Input: part model. Units: mm. Frame: model coordinates. A direction names the side the tool comes from. Round coordinates to 2 decimals unless told otherwise and drop trailing zeros. Loops run counter-clockwise (first coordinate to the right, second up) from the corner with the lowest first, then second, coordinate; pieces in that order, holes last. Notation, with made-up numbers: (-3, 62) -> (16, 62) arc R25 ccw to (16, 74) -> close; hole circle Ø3 at (9.5, 46.5). An arc over 180 degrees is marked (long way). Answer as a JSON object with one key per item and string values.
```python
from build123d import *

# Parameters (mm, degrees)
F1_DEPTH = 550
F2_R     = 6.25
F3_DEPTH = 80.001
F5_DEPTH = 80.001


with BuildPart() as f1:
    # F0 (on Front) → F1 (new body, symmetric)
    with BuildSketch(Plane.XZ):
        with BuildLine():
            ThreePointArc((40, 30), (37.071068, 37.071068), (30, 40))
            Line((30, 40), (-30, 40))
            ThreePointArc((-30, 40), (-37.071068, 37.071068), (-40, 30))
            Line((-40, 30), (-40, -30))
            ThreePointArc((-40, -30), (-37.071068, -37.071068), (-30, -40))
            Line((-30, -40), (30, -40))
            ThreePointArc((30, -40), (37.071068, -37.071068), (40, -30))
            Line((40, -30), (40, 30))
        make_face()
        with BuildLine():
            ThreePointArc((30, 35), (33.535534, 33.535534), (35, 30))
            Line((35, 30), (35, -30))
            ThreePointArc((35, -30), (33.535534, -33.535534), (30, -35))
            Line((30, -35), (-30, -35))
            ThreePointArc((-30, -35), (-33.535534, -33.535534), (-35, -30))
            Line((-35, -30), (-35, 30))
            ThreePointArc((-35, 30), (-33.535534, 33.535534), (-30, 35))
            Line((-30, 35), (30, 35))
        make_face(mode=Mode.SUBTRACT)
    extrude(amount=F1_DEPTH, both=True)

    # F2 (on face) → F3 (cut, through all)
    with BuildSketch(Plane.YZ.offset(40)):
        with Locations((-515, 20)):
            Circle(F2_R)
        with Locations((-515, -20)):
            Circle(F2_R)
        with Locations((-455, 20)):
            Circle(F2_R)
        with Locations((-455, -20)):
            Circle(F2_R)
    extrude(amount=-F3_DEPTH, mode=Mode.SUBTRACT)

    # F4 (on face) → F5 (cut, through all)
    with BuildSketch(Plane.YZ.offset(40)):
        with BuildLine():
            ThreePointArc((450, -5.25), (455.25, 0), (450, 5.25))
            Line((450, 5.25), (300, 5.25))
            ThreePointArc((300, 5.25), (294.75, 0), (300, -5.25))
            Line((300, -5.25), (450, -5.25))
        make_face()
    extrude(amount=-F5_DEPTH, mode=Mode.SUBTRACT)


solid = f1.part
```
1) Contact query for flat-ended pins moving along their axis: P1, Ø14.5, axis at y = -455, z = -20, coming from the +X side; P2, Ø1.5, axis at x = 38, y = 350.5, coming from the -Z side; P3, Ø4, axis at x = -37, y = 352.5, coming from the -Z side; P4, Ø7.5, axis at y = -455, z = -20, coming from the +X side. Output: stop coordinate, or through.
Output:
{"P1": "stops at x = 40", "P2": "stops at z = -36.89", "P3": "stops at z = -38.66", "P4": "passes through"}
2) Section A-A, the plane y = -173. Output: boundary loops of the cut face in (x, z), plus the area to 3 significant figures.
Output:
{"outline": "(-40, -30) arc R10 ccw to (-30, -40) -> (30, -40) arc R10 ccw to (40, -30) -> (40, 30) arc R10 ccw to (30, 40) -> (-30, 40) arc R10 ccw to (-40, 30) -> close; hole (-35, -30) arc R5 ccw to (-30, -35) -> (30, -35) arc R5 ccw to (35, -30) -> (35, 30) arc R5 ccw to (30, 35) -> (-30, 35) arc R5 ccw to (-35, 30) -> close", "area": "1,440 mm^2"}
3) Draft query along X for faces 3 (the face through (0, -8, 40)), 4 (the face through (-40, -8, 0)), 5 (the face through (0, -8, 35)). Return one class per face: +X half, -X half, draft (parallel to the pull), parting line (faces both ways), or undercut.
Output:
{"face 3": "draft", "face 4": "-X half", "face 5": "undercut"}
4) Reachability of faces 1 (the face through (0, -8, -35)), 2 (the face through (-0.2, -550, -35.4)) from +Z, -Z, +X, -X, +Y, -Y: full face, straight path, thin tool, end or side. Return the list, or none.
Output:
{"face 1": "+Y, -Y", "face 2": "+Z, -Z, +X, -X, -Y"}
5) Section B-B, the plane x = -1. Output: boundary loops of the cut face in (y, z).
Output:
{"outline": "(-550, -40) -> (550, -40) -> (550, -35) -> (-550, -35) -> close; (-550, 35) -> (550, 35) -> (550, 40) -> (-550, 40) -> close"}
6) Ray query, probe 1 along X at (y, z) = (-86, -9.5); probe 2 along Z at (x, y) = (36, -515). Return the intervals inside material, ascending.
Output:
{"probe 1": "x = -40 to -35, 35 to 40", "probe 2": "z = -38 to -26.25, -13.75 to 13.75, 26.25 to 38"}
